Can you work these out from the model? Positions are in its coordinate system, mm. Round coordinates to 2 decimals unless told otherwise and drop trailing zeros. Loops run counter-clockwise (first coordinate to the right, second up) from the corner with the lowest first, then second, coordinate; pieces in that order, holes last. Notation, with made-up numbers: (37.25, 39) -> (80.25, 39) arc R27 cw to (80.25, 78) -> close; hole circle Ø11 at (-25.5, 73). An arc over 180 degrees is marked (long way). Answer as a JSON object with one key per item and string values.
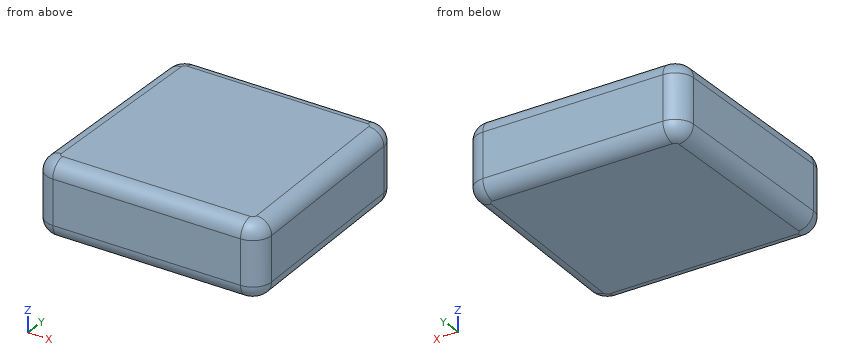
```python
from build123d import *

# Parameters (mm, degrees)
F1_DEPTH = 25.4
F2_R     = 5.08
F3_R     = 5.08


with BuildPart() as f1:
    # F0 (on Top) → F1 (new body)
    with BuildSketch(Plane.XY):
        with BuildLine():
            ThreePointArc((74.904919, -6.080303), (72.95439, -1.765511), (68.560649, 0))
            Line((68.560649, 0), (6.35, 0))
            ThreePointArc((6.35, 0), (1.859872, -1.859872), (0, -6.35))
            Line((0, -6.35), (0, -68.728852))
            ThreePointArc((0, -68.728852), (1.859872, -73.218981), (6.35, -75.078852))
            Line((6.35, -75.078852), (71.212395, -75.078852))
            ThreePointArc((71.212395, -75.078852), (75.796884, -73.122594), (77.556665, -68.459155))
            Line((77.556665, -68.459155), (74.904919, -6.080303))
        make_face()
    extrude(amount=F1_DEPTH)

    # F2
    f2_edges = [f1.edges().sort_by_distance(p)[0] for p in [
        (38.781197, -75.078852, 25.4),
    ]]
    fillet(f2_edges, radius=F2_R)

    # F3
    f3_edges = [f1.edges().sort_by_distance(p)[0] for p in [
        (38.781197, -75.078852, 0),
        (76.230792, -37.269729, 0),
    ]]
    fillet(f3_edges, radius=F3_R)


solid = f1.part
```
Q1. I'm going to push flat-ended pins straight in: pin 1 (1 mm diameter, centred on x = 67, z = 22, fed in from -Y); pin 2 (8 mm diameter, centred on y = -65, z = 15, fed in from +X). Where does each tip first touch, or does it pass through?
Determined:
{"pin 1": "y = -74.94", "pin 2": "x = 77.56"}
Q2. I want a section at A-A, the plane z = 17.5. Write out the boundary of the cut face in (x, y), then the cut area to 3 significant figures.
Determined:
{"outline": "(0, -68.73) arc R6.35 ccw to (6.35, -75.08) -> (71.21, -75.08) arc R6.35 ccw to (77.56, -68.46) -> (74.9, -6.08) arc R6.35 ccw to (68.56, 0) -> (6.35, 0) arc R6.35 ccw to (0, -6.35) -> close", "area": "5,690 mm²"}
Q3. If I drill on L1, parallel to X at y = -19, z = 6.5; L2, parallel to X at y = -61, z = 12.5; L3, parallel to Z at x = 74.5, y = -59, over which ranges is the centre line in solid material (lowest first)? Write a range as [from, to].
Determined:
{"L1": "[0, 75.45]", "L2": "[0, 77.24]", "L3": "[0.62, 24.78]"}
